For this review, take the finished solid that the model builds, in its own axes (mm). Face numbers are marked on the shaded views. A direction names the side the tool comes from. Coordinates: 2 decimals unless noted, no trailing zeros. Write each loop counter-clockwise with the first axis right and the second up, starting at its lowest first coordinate (ties: lowest second). Pieces come first, ordered by that corner, then holes.
1) We need section A-A on z = 4. Write out the cut boundary in (x, y) (3 decimals).
2) We need section D-D on y = 6.25. Write out the cut boundary in (x, z) (3 decimals), then the cut area to 3 significant figures.
3) We need section C-C on x = 10.25. Write out the cut boundary in (y, z).
4) Insertion check: P1, Ø2, axis at x = 2.5, y = 1.5, coming from the +Z side; P2, Ø5, axis at y = 4.5, z = 15.5, coming from the +X side; P3, Ø3, axis at x = 2.5, z = 11.5, coming from the +Y side. Each pin has a flat end and moves straight along its axis. Give the tip position at first contact, or say it passes through.
5) To check wall thickness, follow line 1 along X through (y, z) = (8.25, 4) (3 decimals); line 2 along Y through (x, z) = (7.5, 10.75); line 3 along Z through (x, y) = (7.25, 9). State the ranges of each line that lie inside material, in increasing order.
6) For the marked faces 1 and 2, list the 3-axis set-ups (+Z, -Z, +X, -X, +Y, -Y) from which the entire face can be reached by the end or side of a thin tool; tool diameter is ignored.
7) We need section B-B on y = 13.5. Write out the cut boundary in (x, z) (3 decimals), then the cut area to 3 significant figures.
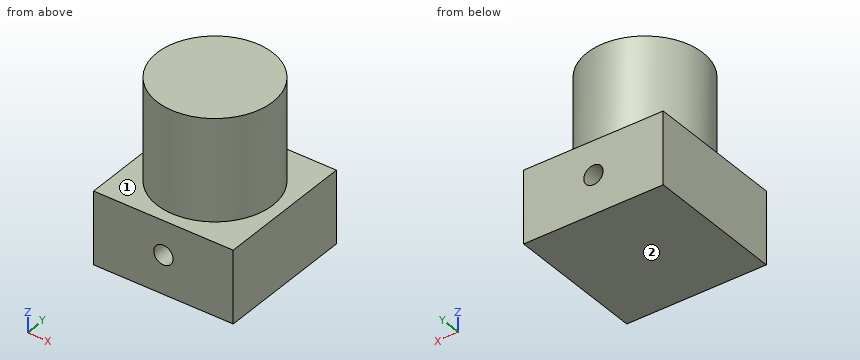
Autodesk Inventor part; units mm, degrees
ref_plane "YZ Plane" through (0, 0, 0) normal (1, 0, 0) x (0, 1, 0)
ref_plane "XZ Plane" through (0, 0, 0) normal (0, 1, 0) x (-1, 0, 0)
ref_plane "XY Plane" through (0, 0, 0) normal (0, 0, 1) x (1, 0, 0)
sketch "Sketch1" plane through (0, 0, 0) normal (0, 0, 1) x (1, 0, 0)
  line L0 (0, 0) -> (14.45, 0)
  line L1 (14.45, 0) -> (14.45, 14.45)
  line L2 (14.45, 14.45) -> (0, 14.45)
  line L3 (0, 14.45) -> (0, 0)
  dimension "d0" = 14.45
  dimension "d1" = 14.45
extrude "Extrusion1" add sketch "Sketch1" along normal blind 7.5
sketch "Sketch6" plane through (0, 0, 7.5) normal (0, 0, 1) x (1, 0, 0)
  line L0 (14.45, 0) -> (14.45, 14.45) construction
  line L1 (14.45, 7.225) -> (0, 7.225) construction
  line L2 (0, 14.45) -> (0, 0) construction
  circle A0 centre (7.225, 7.225) radius 6
  dimension "d14" = 12
sketch "Sketch7" plane through (0, 0, 0) normal (-1, 0, 0) x (0, 0, 1)
  line L0 (0, 14.45) -> (0, 0)
  line L1 (0, 0) -> (7.5, 0)
  line L2 (7.5, 14.45) -> (7.5, 0)
  line L3 (0, 14.45) -> (7.5, 14.45)
  dimension "d15" = 7.5
extrude "Extrusion4" add sketch "Sketch6" along normal blind 10.5
sketch "Sketch8" plane through (0, 14.45, 0) normal (0, 1, 0) x (1, 0, 0)
  line L0 (14.45, 0) -> (0, 0)
  line L1 (0, 0) -> (14.45, 0) construction
  line L2 (7.225, 0) -> (7.225, -5) construction
  line L3 (7.225, -5) -> (9.4124, -5) construction
  circle A0 centre (7.225, -4) radius 1
  dimension "d18" = 5
  dimension "d19" = 2
extrude "Extrusion5" cut sketch "Sketch8" against normal up to surface (14.45 mm away)
sketch "Sketch10" plane through (0, 14.45, 0) normal (0, 1, 0) x (1, 0, 0)
  circle A0 centre (7.225, -4) radius 1
  line L0 (7.225, -4) -> (7.225, -117.6084)
  line L1 (-3.4196, -20.1658) -> (-107.1714, -68.5461)
  line L2 (1.225, -18) -> (13.225, -18)
  line L3 (13.225, -18) -> (159.9004, -86.3959)
  point P0 (0, 0)
  dimension "d22" = 130
properties part number "HDzero runcam nano spacer"
Result:
1. outline: (0, 0) - (6.225, 0) - (6.225, 14.45) - (0, 14.45) - close; (8.225, 0) - (14.45, 0) - (14.45, 14.45) - (8.225, 14.45) - close
2. outline: (0, 0) - (14.45, 0) - (14.45, 7.5) - (13.145, 7.5) - (13.145, 18) - (1.305, 18) - (1.305, 7.5) - (0, 7.5) - close; hole circle Ø2 at (7.225, 4)
2. area: 230 mm2
3. outline: (0, 0) - (14.45, 0) - (14.45, 7.5) - (12.41, 7.5) - (12.41, 18) - (2.04, 18) - (2.04, 7.5) - (0, 7.5) - close
4. P1: stops at z = 7.5
4. P2: stops at x = 13.22
4. P3: stops at y = 12.28
5. line 1: x = 0 to 6.225, 8.225 to 14.45
5. line 2: y = 1.23 to 13.22
5. line 3: z = 0 to 3, 5 to 18
6. face 1: +Z
6. face 2: -Z, +X, -X, +Y, -Y
7. outline: (0, 0) - (14.45, 0) - (14.45, 7.5) - (0, 7.5) - close; hole circle Ø2 at (7.225, 4)
7. area: 105 mm2
